Check sheet for the drawn part. Datum: minimum x, y, z corner. Units: mm. A direction names the side the tool comes from. Coordinates: 2 decimals unless noted, no trailing zeros. Write each loop counter-clockwise with the first axis right and the second up, starting at its lowest first coordinate (ties: lowest second). Pieces come first, ordered by that corner, then holes. Notation, with made-up numbers: (-26, -0.5) -> (30, -0.5) arc R21 cw to (30, 7.5) -> close; hole circle Ø11 at (73, 87.25). An arc over 180 degrees is marked (long way). Answer in a Markdown table with one row per item. Add a question column.
Q1. Section check D-D, the plane z = 68.5. Record the boundary of the cut face in (x, y), and give its area (3 significant figures).
Q2. Section check C-C, the plane y = 39.5. Record the boundary of the cut face in (x, z).
Q3. Thickness scan on line 1 (X direction, y = 16.5, z = 19.5); line 2 (Z direction, x = 88, y = 36.5); line 3 (X direction, y = 10.5, z = 14). Record the ranges inside material, lowest first.
Q4. Tool access check on the marked faces 1 and 2. Record the directions out of +Z, -Z, +X, -X, +Y, -Y that give a thin tool (end or side, any length) a straight path to the whole face; none if there is none.
Q5. Release check for a two-part mould opening along X. For the marked faces 3, 4, 5 and 6 record: pulls with the +X half, pulls with the -X half, needs draft (parallel to the pull), parting line crosses it, or undercut.
Q6. Gauge pin test, flat ends, axial feed: P1, Ø0.6, axis at x = 1, z = 23.5, coming from the +Y side; P2, Ø12, axis at x = 76, z = 42.5, coming from the -Y side; P3, Ø2, axis at y = 1, z = 21.5, coming from the -X side; P4, Ø1.6, axis at x = 1, y = 11.5, coming from the +Z side. Record the tip position at first contact, or that the pin passes through.
Q7. Section check A-A, the plane z = 13. Record the boundary of the cut face in (x, y), and give its area (3 significant figures).
Q8. Section check B-B, the plane x = 46. Record the boundary of the cut face in (y, z).
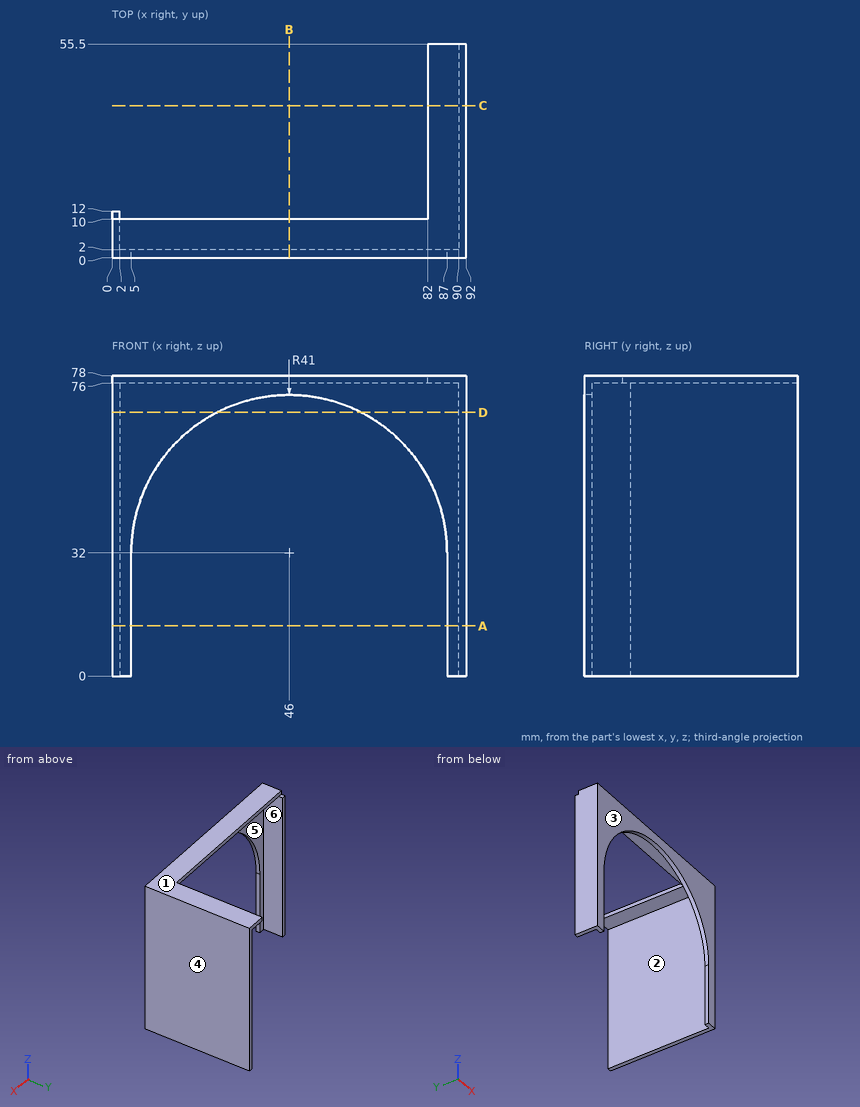
Calculated:
| question | item | result |
|---|---|---|
| 1 | outline | (0, 0) -> (27.33, 0) -> (27.33, 2) -> (2, 2) -> (2, 12) -> (0, 12) -> close; (64.67, 0) -> (92, 0) -> (92, 55.5) -> (90, 55.5) -> (90, 2) -> (64.67, 2) -> close |
| 1 | area | 236 mm² |
| 2 | outline | (82, 76) -> (90, 76) -> (90, 0) -> (92, 0) -> (92, 78) -> (82, 78) -> close |
| 3 | line 1 | x = 90 to 92 |
| 3 | line 2 | z = 76 to 78 |
| 3 | line 3 | x = 0 to 2, 90 to 92 |
| 4 | face 1 | +Z, +X, -X, +Y, -Y |
| 4 | face 2 | -Z, +Y |
| 5 | face 3 | needs draft |
| 5 | face 4 | pulls with the +X half |
| 5 | face 5 | undercut |
| 5 | face 6 | undercut |
| 6 | P1 | stops at y = 12 |
| 6 | P2 | passes through |
| 6 | P3 | stops at x = 0 |
| 6 | P4 | stops at z = 76 |
| 7 | outline | (0, 0) -> (5, 0) -> (5, 2) -> (2, 2) -> (2, 12) -> (0, 12) -> close; (87, 0) -> (92, 0) -> (92, 55.5) -> (90, 55.5) -> (90, 2) -> (87, 2) -> close |
| 7 | area | 147 mm² |
| 8 | outline | (0, 73) -> (2, 73) -> (2, 76) -> (10, 76) -> (10, 78) -> (0, 78) -> close |
